Design review of the part built by this model. Coordinates are the model's own, in mm. Face numbers are marked on the shaded views. A direction names the side the tool comes from. Coordinates: 2 decimals unless noted, no trailing zeros. Loops run counter-clockwise (first coordinate to the right, second up) from the corner with the lowest first, then second, coordinate; pieces in that order, holes last.
from build123d import *

# Parameters (mm, degrees)
F3_DEPTH = 3


with BuildPart() as f1:
    # F0 (on Front) → F1 (revolve)
    with BuildSketch(Plane.XZ):
        Polygon((28.186478, 0), (0, 0), (0, -4.948771), (25.389344, -4.948771), align=None)
    revolve(axis=Axis((0, 0, -2.474385), (0, 0, 1)))

    # F2 (on Top) → F3 (join)
    with BuildSketch(Plane.XY):
        Polygon((-36.147542, -7.10041), (-36.147542, -10.543033), (0, -10.543033), (36.147542, -10.543033), (36.147542, -7.10041), (31.198772, -7.10041), (31.198772, 0), (31.198772, 7.10041), (36.147542, 7.10041), (36.147542, 10.543033), (0, 10.543033), (-36.147542, 10.543033), (-36.147542, 7.10041), (-31.198772, 7.10041), (-31.198772, 0), (-31.198772, -7.10041), align=None)
    extrude(amount=F3_DEPTH)


solid = f1.part
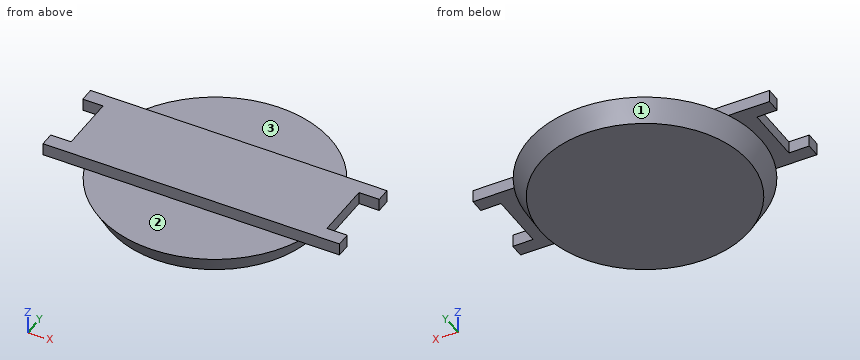
Q1. For line 1 (Z direction, x = -6, y = 11); line 2 (Y direction, x = -23, z = 0.5); line 3 (Z direction, x = -28, y = -3.5), list the stretches that pass through material, from the lowest coordinate up.
Q2. Take a section at B-B, the plane y = 0. Write out the cut boundary in (x, z).
Q3. Clearance check with flat-ended pins moving along their axes: pin 1 Ø1.5 at (x, z) = (-10, 1.5) entering from +Y; pin 2 Ø4 at (x, z) = (26, -2.5) entering from -Y; pin 3 Ø3.5 at (x, z) = (-15.5, 1.5) entering from -Y. State where each tip first meets the part, or that it passes through.
Q4. Take a section at A-A, the plane x = 0. Write out the cut boundary in (y, z), then the cut area to 3 significant figures.
Q5. Machinability: for the marked faces 1, 2 and 3, which of the approach directions +Z, -Z, +X, -X, +Y, -Y give a long, thin tool a straight path to every point of the face, cutting with its end or side? Answer none if there is none.
Q6. Take a section at C-C, the plane z = -2. Write out the cut boundary in (x, y).
Entries:
1. line 1: z = -4.95 to 0
1. line 2: y = -10.54 to 10.54
1. line 3: z = 0 to 3
2. outline: (-31.2, 0) - (-28.19, 0) - (-25.39, -4.95) - (25.39, -4.95) - (28.19, 0) - (31.2, 0) - (31.2, 3) - (-31.2, 3) - close
3. pin 1: stops at y = 10.54
3. pin 2: stops at y = -12.59
3. pin 3: stops at y = -24.11
4. outline: (-28.19, 0) - (-25.39, -4.95) - (25.39, -4.95) - (28.19, 0) - (10.54, 0) - (10.54, 3) - (-10.54, 3) - (-10.54, 0) - close
4. area: 328 mm2
5. face 1: -Z
5. face 2: +Z, +X, -X, -Y
5. face 3: +Z, +X, -X, +Y
6. outline: circle Ø54.11 at (0, 0)
